Source: CAD feature listing. Evaluate the final solid. Frame: model axes, mm. Face numbers are marked on the shaded views. A direction names the side the tool comes from. Give positions to 0.01 mm unless a question says otherwise; leave off trailing zeros. Write each loop counter-clockwise with the first axis right and the second up, starting at its lowest first coordinate (ties: lowest second). Pieces come first, ordered by that corner, then holes.
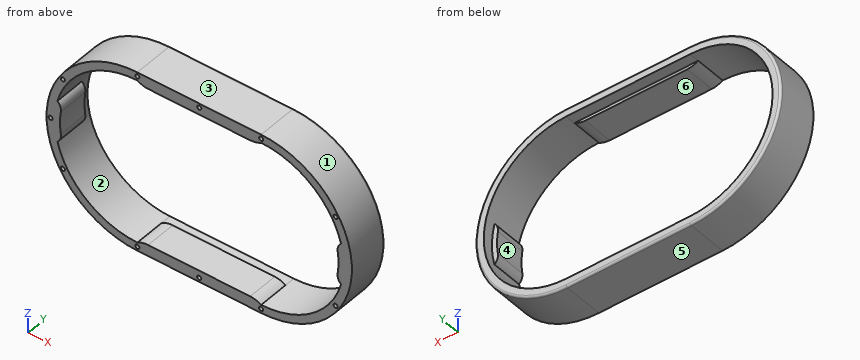
```python
from build123d import *

# Parameters (mm, degrees)
BOSS_EXTRUDE1_DEPTH = 20
SHELL1_T            = -4
SKETCH3_W           = 60
SKETCH3_H           = 1.5
BOSS_EXTRUDE2_DEPTH = 15
BOSS_EXTRUDE3_DEPTH = 15
FILLET2_R           = 10
BOSS_EXTRUDE5_DEPTH = 15
FILLET5_R           = 5
FILLET6_R           = 1
SKETCH7_R           = 1
CUT_EXTRUDE1_DEPTH  = 3


with BuildPart() as part:
    # Sketch1 → Boss-Extrude1 (new body)
    with BuildSketch(Plane(origin=(0, 0, 0), x_dir=(1, 0, 0), z_dir=(0, 1, 0))):
        with BuildLine():
            Line((0, 0), (60, 0))
            ThreePointArc((60, 0), (104, 44), (60, 88))
            Line((60, 88), (0, 88))
            ThreePointArc((0, 88), (-44, 44), (0, 0))
        make_face()
    extrude(amount=BOSS_EXTRUDE1_DEPTH)

    # Shell1
    shell1_openings = [part.faces().sort_by_distance(p)[0] for p in [
        (30, 20, -44),
        (30, 0, -44),
    ]]
    offset(amount=SHELL1_T, openings=shell1_openings, kind=Kind.INTERSECTION)

    # Sketch3 → Boss-Extrude2 (add)
    with BuildSketch(Plane.XZ):
        with Locations((30, -4.75)):
            Rectangle(SKETCH3_W, SKETCH3_H)
    extrude(amount=-BOSS_EXTRUDE2_DEPTH)

    # Sketch5 → Boss-Extrude3 (add)
    with BuildSketch(Plane.XZ):
        Polygon((0, -84), (0, -82.5), (60.003782522, -82.5), (60, -84), align=None)
    extrude(amount=-BOSS_EXTRUDE3_DEPTH)

    # Fillet2
    # the kernel refuses this fillet: 10 mm, written as the material it takes off along each edge
    with BuildSketch(Plane(origin=(60, -13.169567191, -5.5), x_dir=(0, 0, 1), z_dir=(0, 1, 0)), Plane(origin=(0, -13.169567191, -82.5), x_dir=(0, 0, -1), z_dir=(0, 1, 0))) as fillet2_piece_1:
        with BuildLine():
            CenterArc((10, -5.267826876), FILLET2_R, 148.211669383, 31.788330617)
            Line((0, -5.267826876), (-0.2, -5.267826876))
            Line((-0.2, -5.267826876), (-0.2, 0))
            Line((-0.2, 0), (0, 0.2))
            ThreePointArc((0, 0.2), (0.75, 0.2), (1.33, 0.105356538))
            Line((1.33, 0.105356538), (1.5, 0))
        make_face()
    extrude(amount=41.339134382, mode=Mode.SUBTRACT)
    with BuildSketch(Plane(origin=(60.003782522, -13.179023495, -82.5), x_dir=(-1, 0, 0), z_dir=(0, 1, 0))) as fillet2_piece_2:
        with BuildLine():
            CenterArc((5.271609398, -10), FILLET2_R, 90, 31.788330617)
            Line((0.003782522, -1.5), (-0.101574016, -1.33))
            ThreePointArc((-0.101574016, -1.33), (-0.198108103, -0.750504335), (-0.199999364, -0.000504335))
            Line((-0.199999364, -0.000504335), (0, 0.2))
            Line((0, 0.2), (5.271609398, 0.2))
            Line((5.271609398, 0.2), (5.271609398, 0))
        make_face()
    extrude(amount=41.358046991, mode=Mode.SUBTRACT)
    with BuildSketch(Plane(origin=(0, -13.169567191, -5.5), x_dir=(1, 0, 0), z_dir=(0, 1, 0))) as fillet2_piece_3:
        with BuildLine():
            CenterArc((5.267826876, -10), FILLET2_R, 90, 31.788330617)
            Line((0, -1.5), (-0.105356538, -1.33))
            ThreePointArc((-0.105356538, -1.33), (-0.2, -0.75), (-0.2, 0))
            Line((-0.2, 0), (0, 0.2))
            Line((0, 0.2), (5.267826876, 0.2))
            Line((5.267826876, 0.2), (5.267826876, 0))
        make_face()
    extrude(amount=41.339134382, mode=Mode.SUBTRACT)

    # Sketch8 → Boss-Extrude5 (add)
    with BuildSketch(Plane.XZ):
        with BuildLine():
            Line((96.142080737, -34), (98.729833462, -34))
            ThreePointArc((98.729833462, -34), (100, -44), (98.729833462, -54))
            Line((98.729833462, -54), (96.142080737, -54))
            ThreePointArc((96.142080737, -54), (97.5, -44), (96.142080737, -34))
        make_face()
        with BuildLine():
            Line((-36.142080737, -54), (-38.729833462, -54))
            ThreePointArc((-38.729833462, -54), (-40, -44), (-38.729833462, -34))
            Line((-38.729833462, -34), (-36.142080737, -34))
            ThreePointArc((-36.142080737, -34), (-37.5, -44), (-36.142080737, -54))
        make_face()
    extrude(amount=-BOSS_EXTRUDE5_DEPTH)

    # Fillet5
    # the kernel refuses this fillet: 5 mm, written as the material it takes off along each edge
    with BuildSketch(Plane(origin=(96.142080737, -11.460527233, -34), x_dir=(1, 0, 0), z_dir=(0, 1, 0)), Plane(origin=(-36.142080737, -11.460527233, -54), x_dir=(-1, 0, 0), z_dir=(0, 1, 0))) as fillet5_piece_1:
        with BuildLine():
            CenterArc((5.895743435, 3.749292929), FILLET5_R, 171.542516957, 57.035612676)
            Line((0.950117062, 4.484670231), (0.851204534, 4.499377777))
            ThreePointArc((0.851204534, 4.499377777), (0.445822951, 2.248528932), (-0.096378882, 0.026666667))
            Line((-0.096378882, 0.026666667), (0, -0.1))
            ThreePointArc((0, -0.1), (1.293876363, -0.1), (2.521592911, -0.074985859))
            Line((2.521592911, -0.074985859), (2.587752725, 0))
        make_face()
    extrude(amount=37.921054465, mode=Mode.SUBTRACT)
    with BuildSketch(Plane(origin=(96.142080737, -11.460527233, -54), x_dir=(1, 0, 0), z_dir=(0, 1, 0)), Plane(origin=(-36.142080737, -11.460527233, -34), x_dir=(-1, 0, 0), z_dir=(0, 1, 0))) as fillet5_piece_2:
        with BuildLine():
            CenterArc((5.895743435, -3.749292929), FILLET5_R, 131.421870366, 57.035612676)
            Line((0.950117062, -4.484670231), (0.851204534, -4.499377777))
            ThreePointArc((0.851204534, -4.499377777), (0.445822951, -2.248528932), (-0.096378882, -0.026666667))
            Line((-0.096378882, -0.026666667), (0, 0.1))
            ThreePointArc((0, 0.1), (1.293876363, 0.1), (2.521592911, 0.074985859))
            Line((2.521592911, 0.074985859), (2.587752725, 0))
        make_face()
    extrude(amount=37.921054465, mode=Mode.SUBTRACT)

    # Fillet6
    fillet6_edges = [part.edges().sort_by_distance(p)[0] for p in [
        (104, 20, -44),
        (30, 20, -88),
        (-44, 20, -44),
        (30, 20, 0),
    ]]
    fillet(fillet6_edges, radius=FILLET6_R)

    # Sketch7 → Cut-Extrude1 (cut)
    with BuildSketch(Plane.XZ):
        with Locations(Location((-42, -44, 0), (0, 0, 270))):
            Circle(SKETCH7_R)
        with Locations(Location((-36.105117767, -22, 0), (0, 0, 270))):
            Circle(SKETCH7_R)
        with Locations(Location((-36.105117767, -66, 0), (0, 0, 90))):
            Circle(SKETCH7_R)
        with Locations(Location((0, -2, 0), (0, 0, 270))):
            Circle(SKETCH7_R)
        with Locations(Location((30, -2, 0), (0, 0, 270))):
            Circle(SKETCH7_R)
        with Locations(Location((0, -86, 0), (0, 0, 270))):
            Circle(SKETCH7_R)
        with Locations(Location((30, -86, 0), (0, 0, 270))):
            Circle(SKETCH7_R)
        with Locations(Location((96.105117767, -22, 0), (0, 0, 90))):
            Circle(SKETCH7_R)
        with Locations(Location((96.105117767, -66, 0), (0, 0, 270))):
            Circle(SKETCH7_R)
        with Locations(Location((60, -86, 0), (0, 0, 90))):
            Circle(SKETCH7_R)
        with Locations(Location((60, -2, 0), (0, 0, 90))):
            Circle(SKETCH7_R)
    extrude(amount=-CUT_EXTRUDE1_DEPTH, mode=Mode.SUBTRACT)


solid = part.part
```
1. Section query A-A (y = 7). Return loops of the section in (x, z), plus the area to 3 significant figures.
2. Pull-direction query (X, two-part tool) for the marked faces 1, 2, 3 and 4; classes: pulls with the +X half, pulls with the -X half, needs draft (parallel to the pull), parting line crosses it, or undercut.
3. Access query for the marked faces 5 and 6. Directions: +Z, -Z, +X, -X, +Y, -Y. A direction counts if a zero-diameter tool reaches every point of the face in a straight line with its end or side. Return the directions, or none.
4. Line query: probe 1 along X at (y, z) = (0.7, -66); probe 2 along Z at (x, y) = (60.5, 14); probe 3 along Z at (x, y) = (7, 7). Output: solid intervals per line, ascending.
5. Pin query (flat end, axial travel): P1, Ø4, axis at x = -11, y = 15, coming from the +Z side; P2, Ø1, axis at y = 4.5, z = -14.5, coming from the +X side; P3, Ø1.6, axis at x = 0, z = -86, coming from the -Y side. Return the tip coordinate at first contact, or that it passes through.
The answers:
1. outline: (0, -88) - (60, -88) arc R44 ccw to (60, 0) - (0, 0) arc R44 ccw to start; hole (-38.73, -54) arc R40 ccw to (0, -84) arc R10 cw to (5.27, -82.5) - (54.73, -82.5) arc R10 cw to (60, -84) arc R40 ccw to (98.73, -54) arc R5 cw to (97.09, -49.52) arc R37.5 ccw to (97.09, -38.48) arc R5 cw to (98.73, -34) arc R40 ccw to (60, -4) arc R10 cw to (54.73, -5.5) - (5.27, -5.5) arc R10 cw to (0, -4) arc R40 ccw to (-38.73, -34) arc R5 cw to (-37.09, -38.48) arc R37.5 ccw to (-37.09, -49.52) arc R5 cw to start
1. area: 1,790 mm2
2. face 1: pulls with the +X half
2. face 2: undercut
2. face 3: needs draft
2. face 4: undercut
3. face 5: -Z, +X, -X, +Y, -Y
3. face 6: +Y, -Y
4. probe 1: x = -38.11 to -37.11, -35.11 to -33.41, 93.41 to 95.11, 97.11 to 98.11
4. probe 2: z = -88 to -84, -4 to 0
4. probe 3: z = -88 to -82.5, -5.5 to 0
5. P1: stops at z = -0.93
5. P2: stops at x = 93.09
5. P3: stops at y = 3
